```python
from build123d import *

# Parameters (mm, degrees)
EXTRUDE1_DEPTH = 6


with BuildPart() as part:
    # Sketch1 → Extrude1 (new body, symmetric)
    with BuildSketch(Plane(origin=(0, 0, 0), x_dir=(0, 0, -1), z_dir=(1, 0, 0))):
        with BuildLine():
            Line((105.67734259, 13.838708831), (302.152337132, 2.666129904))
            Line((302.152337132, 2.666129904), (306, 2.447331999))
            Line((306, 2.447331999), (306, 0))
            Line((306, 0), (100, 0))
            Line((100, 0), (100, 14))
            ThreePointArc((100, 14), (102.839816619, 13.959669075), (105.67734259, 13.838708831))
        make_face()
    extrude1 = extrude(amount=EXTRUDE1_DEPTH, both=True)

    # Mirror1: Extrude1 across plane
    add(extrude1.mirror(Plane(origin=(6, 0, -306), x_dir=(0, 0, 1), z_dir=(0, 1, 0))))


solid = part.part
```
The listing builds one solid part. Answer for the finished solid, in the listing's coordinates (mm). Round coordinates to 2 decimals unless told otherwise and drop trailing zeros. Write each loop counter-clockwise with the first axis right and the second up, starting at its lowest first coordinate (ties: lowest second). Pieces come first, ordered by that corner, then holes. Notation, with made-up numbers: (-14.5, 3.25) -> (43.5, 3.25) arc R18 ccw to (43.5, 29.25) -> close; hole circle Ø6 at (25, 46.25). An arc over 180 degrees is marked (long way). Use CSV: the item, a comma, the result in double quotes. Start each with the question number.
(1) Consider L1, parallel to Y at x = 4.5, z = -276.5; L2, parallel to Y at x = 1.75, z = -227. Determine where each line is inside the solid, lowest interval first. Write a range as from..to.
(2) Each of these flat-tipped pins is pushed along its axis until it touches: pin 1 (5 mm diameter, centred on x = 0, z = -153.5, fed in from -Y); pin 2 (5 mm diameter, centred on x = -4, z = -188.5, fed in from +Y). Where does it stop, or does it pass through?
(3) Section C-C on y = -4.5 is taken. Give the vertices of the cut face in (x, z).
(4) Section B-B on z = -239 is taken. Give the vertices of the cut face in (x, y), then the cut area to 3 significant figures.
(5) Section A-A on x = 2 is taken. Give the vertices of the cut face in (y, z), then the cut area to 3 significant figures.
A:
1,L1,"y = -4.12..4.12"
1,L2,"y = -6.94..6.94"
2,pin 1,"stops at y = -11.26"
2,pin 2,"stops at y = 9.27"
3,outline,"(-6, -269.9) -> (6, -269.9) -> (6, -100) -> (-6, -100) -> close"
4,outline,"(-6, -6.26) -> (6, -6.26) -> (6, 6.26) -> (-6, 6.26) -> close"
4,area,"150 mm²"
5,outline,"(-14, -100) arc R100 ccw to (-13.84, -105.68) -> (-2.45, -306) -> (2.45, -306) -> (13.84, -105.68) arc R100 ccw to (14, -100) -> close"
5,area,"3,420 mm²"
